Could you check a few things on this drawing? It's one solid part, dimensions in mm from its lowest x, y, z. A direction names the side the tool comes from. Give positions to 0.01 mm unless a question says otherwise; leave off trailing zeros. Order: outer loops, then holes, each group sorted by start corner. A loop starts at its lowest first (then second) coordinate and runs counter-clockwise, first axis right, second up. Notation, with made-up numbers: (54, 2) - (113, 2) arc R18 cw to (113, 19) - close; hole circle Ø9 at (-4.75, 69). An arc over 180 degrees is marked (long way). Return JSON: item names as keys, results as strings.
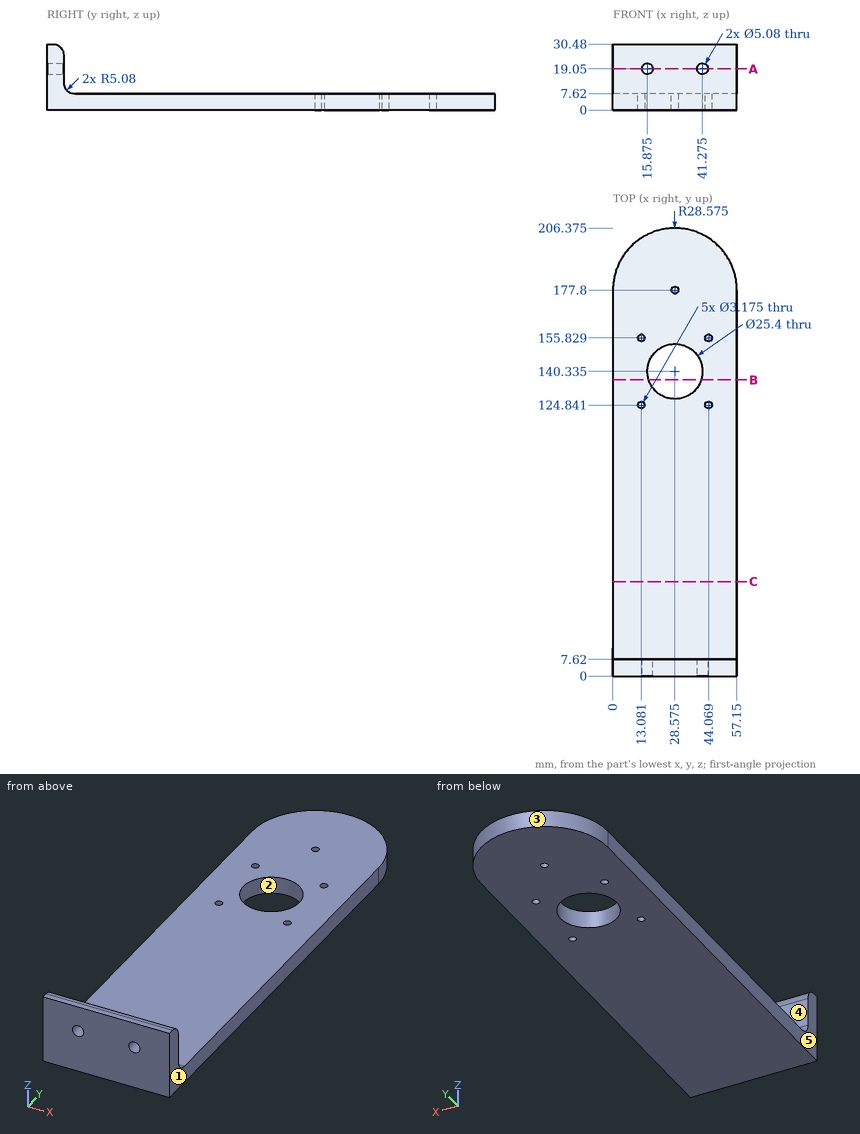
1. If I drill on L1, parallel to X at y = 177.8, z = 6; L2, parallel to Y at x = 45.5, z = 7.5; L3, parallel to Z at x = 10.5, y = 67, over which ranges is the centre line in solid material (lowest first)? Write a range as [from, to].
Checks:
{"L1": "[0, 26.99], [30.16, 57.15]", "L2": "[0, 124.15], [125.53, 155.14], [156.52, 200.82]", "L3": "[0, 7.62]"}
2. On a 3-axis mill with a long thin cutter (end or side, diameter ignored), from which of +Z, -Z, +X, -X, +Y, -Y can I reach the whole of each face in a straight line? I mean the marked faces 4 and 5. Say none if no direction works.
Checks:
{"face 4": "+Z, +X, -X, +Y", "face 5": "+Z, -Z, -X, +Y, -Y"}
3. Suppose I cut it at B-B (y = 136.5). List the corners of the cut face in (x, z) for me, plus the area to 3 significant figures.
Checks:
{"outline": "(0, 0) - (16.47, 0) - (16.47, 7.62) - (0, 7.62) - close; (40.68, 0) - (57.15, 0) - (57.15, 7.62) - (40.68, 7.62) - close", "area": "251 mm^2"}
4. Thinking about a two-plate mould opening in X: for the marked faces 1, 2 and 3, which applies, +X half, -X half, draft (parallel to the pull), parting line (faces both ways), or undercut?
Checks:
{"face 1": "+X half", "face 2": "undercut", "face 3": "parting line"}
5. For pin 1 Ø3.5 at (x, y) = (13.081, 124.841) entering from +Z; pin 2 Ø14 at (x, z) = (23, 16) entering from +Y; pin 3 Ø8 at (x, z) = (46, 11) entering from +Y, each with a flat end and sliding along its axis, tell me the tip position at first contact or that it passes through.
Checks:
{"pin 1": "z = 7.62", "pin 2": "y = 9.22", "pin 3": "y = 201.94"}
6. Suppose I cut it at C-C (y = 43.5). List the corners of the cut face in (x, z) for me, plus the area to 3 significant figures.
Checks:
{"outline": "(0, 0) - (57.15, 0) - (57.15, 7.62) - (0, 7.62) - close", "area": "435 mm^2"}
7. Suppose I cut it at A-A (z = 19.05). List the corners of the cut face in (x, y) for me (3 decimals).
Checks:
{"outline": "(0, 0) - (13.335, 0) - (13.335, 7.62) - (0, 7.62) - close; (18.415, 0) - (38.735, 0) - (38.735, 7.62) - (18.415, 7.62) - close; (43.815, 0) - (57.15, 0) - (57.15, 7.62) - (43.815, 7.62) - close"}
